from build123d import *

# Parameters (mm, degrees)
ESTRUSIONE_ESTRUSIONE1_DEPTH  = 10
TAGLIO_ESTRUSIONE1_DEPTH      = 3
SCHIZZO4_W                    = 80
SCHIZZO4_H                    = 5
ESTRUSIONE_ESTRUSIONE2_DEPTH  = 35
ESTRUSIONE_ESTRUSIONE4_DEPTH  = 80
SCHIZZO7_W                    = 80
SCHIZZO7_H                    = 5
ESTRUSIONE_ESTRUSIONE5_DEPTH  = 7
TAGLIO_ESTRUSIONE2_REACH      = 112.369
SCHIZZO8_R                    = 1.5
RACCORDO1_R                   = 5
RACCORDO2_R                   = 5
TAGLIO_ESTRUSIONE3_DEPTH      = 111.368700273
TAGLIO_ESTRUSIONE3_DEPTH_BACK = 10
SCHIZZO11_R                   = 4
TAGLIO_ESTRUSIONE4_DEPTH      = 3
SCHIZZO12_W                   = 12
SCHIZZO12_H                   = 12
ESTRUSIONE_ESTRUSIONE6_DEPTH  = 40
SCHIZZO13_R                   = 1.5
TAGLIO_ESTRUSIONE5_DEPTH      = 111.368700273
SCHIZZO14_R                   = 4
TAGLIO_ESTRUSIONE6_DEPTH      = 10


with BuildPart() as part:
    # Schizzo1 → Estrusione-Estrusione1 (new body)
    with BuildSketch(Plane.XY):
        with BuildLine():
            Line((-76.016095604, 20), (76.016095604, 20))
            ThreePointArc((76.016095604, 20), (92.5, 0), (76.016095604, -20))
            Line((76.016095604, -20), (-76.016095604, -20))
            ThreePointArc((-76.016095604, -20), (-92.5, 0), (-76.016095604, 20))
        make_face()
    extrude(amount=ESTRUSIONE_ESTRUSIONE1_DEPTH)

    # Schizzo3 → Taglio-Estrusione1 (cut)
    with BuildSketch(Plane.XY.offset(10)):
        with BuildLine():
            Line((-75.5, -15), (75.5, -15))
            ThreePointArc((75.5, -15), (87.5, 0), (75.5, 15))
            Line((75.5, 15), (-75.5, 15))
            ThreePointArc((-75.5, 15), (-87.5, 0), (-75.5, -15))
        make_face()
    extrude(amount=-TAGLIO_ESTRUSIONE1_DEPTH, mode=Mode.SUBTRACT)

    # Schizzo4 → Estrusione-Estrusione2 (add)
    with BuildSketch(Plane.XY.offset(10)):
        with Locations((0, -17.5)):
            Rectangle(SCHIZZO4_W, SCHIZZO4_H)
    estrusione_estrusione2 = extrude(amount=ESTRUSIONE_ESTRUSIONE2_DEPTH)

    # Schizzo6 → Estrusione-Estrusione4 (add)
    with BuildSketch(Plane(origin=(40, 0, 0), x_dir=(0, 0, -1), z_dir=(1, 0, 0))):
        Polygon((-40, -15), (-40, -12.81), (-7, -15), align=None)
    estrusione_estrusione4 = extrude(amount=-ESTRUSIONE_ESTRUSIONE4_DEPTH)

    # Schizzo7 → Estrusione-Estrusione5 (add)
    with BuildSketch(Plane(origin=(0, -15, 0), x_dir=(1, 0, 0), z_dir=(0, 1, 0))):
        with Locations((0, -42.5)):
            Rectangle(SCHIZZO7_W, SCHIZZO7_H)
    estrusione_estrusione5 = extrude(amount=ESTRUSIONE_ESTRUSIONE5_DEPTH)

    # Taglio-Estrusione2: up to this plane
    taglio_estrusione2_end = Plane(origin=(-40, -12.81, 40), z_dir=(1.4576135341627736e-15, 0.9978051809344605, -0.0662179801892863))
    # Schizzo8 → Taglio-Estrusione2 (cut, up to the surface)
    with BuildSketch(Plane.XZ.offset(20), mode=Mode.PRIVATE) as taglio_estrusione2_sk1:
        with Locations(Location((-30, 13, 0), (0, 0, 270))):
            Circle(SCHIZZO8_R)
    taglio_estrusione2_tool1 = split(extrude(taglio_estrusione2_sk1.sketch, amount=-TAGLIO_ESTRUSIONE2_REACH, mode=Mode.PRIVATE), bisect_by=taglio_estrusione2_end, keep=Keep.BOTH, mode=Mode.PRIVATE)
    add(taglio_estrusione2_tool1.solids().sort_by_distance((-30, -20, 13))[0], mode=Mode.SUBTRACT)
    # Schizzo8 → Taglio-Estrusione2 (cut, up to the surface)
    with BuildSketch(Plane.XZ.offset(20), mode=Mode.PRIVATE) as taglio_estrusione2_sk2:
        with Locations(Location((-30, 32, 0), (0, 0, 270))):
            Circle(SCHIZZO8_R)
    taglio_estrusione2_tool2 = split(extrude(taglio_estrusione2_sk2.sketch, amount=-TAGLIO_ESTRUSIONE2_REACH, mode=Mode.PRIVATE), bisect_by=taglio_estrusione2_end, keep=Keep.BOTH, mode=Mode.PRIVATE)
    add(taglio_estrusione2_tool2.solids().sort_by_distance((-30, -20, 32))[0], mode=Mode.SUBTRACT)
    # Schizzo8 → Taglio-Estrusione2 (cut, up to the surface)
    with BuildSketch(Plane.XZ.offset(20), mode=Mode.PRIVATE) as taglio_estrusione2_sk3:
        with Locations(Location((30, 13, 0), (0, 0, 270))):
            Circle(SCHIZZO8_R)
    taglio_estrusione2_tool3 = split(extrude(taglio_estrusione2_sk3.sketch, amount=-TAGLIO_ESTRUSIONE2_REACH, mode=Mode.PRIVATE), bisect_by=taglio_estrusione2_end, keep=Keep.BOTH, mode=Mode.PRIVATE)
    add(taglio_estrusione2_tool3.solids().sort_by_distance((30, -20, 13))[0], mode=Mode.SUBTRACT)
    # Schizzo8 → Taglio-Estrusione2 (cut, up to the surface)
    with BuildSketch(Plane.XZ.offset(20), mode=Mode.PRIVATE) as taglio_estrusione2_sk4:
        with Locations(Location((30, 32, 0), (0, 0, 270))):
            Circle(SCHIZZO8_R)
    taglio_estrusione2_tool4 = split(extrude(taglio_estrusione2_sk4.sketch, amount=-TAGLIO_ESTRUSIONE2_REACH, mode=Mode.PRIVATE), bisect_by=taglio_estrusione2_end, keep=Keep.BOTH, mode=Mode.PRIVATE)
    add(taglio_estrusione2_tool4.solids().sort_by_distance((30, -20, 32))[0], mode=Mode.SUBTRACT)

    # Specchia1: Estrusione-Estrusione2, Estrusione-Estrusione4, Estrusione-Estrusione5 across plane
    add(estrusione_estrusione2.mirror(Plane.ZX))
    add(estrusione_estrusione4.mirror(Plane.ZX))
    add(estrusione_estrusione5.mirror(Plane.ZX))

    # Raccordo1
    raccordo1_edges = [part.edges().sort_by_distance(p)[0] for p in [
        (0, -20, 45),
    ]]
    fillet(raccordo1_edges, radius=RACCORDO1_R)

    # Raccordo2
    raccordo2_edges = [part.edges().sort_by_distance(p)[0] for p in [
        (0, 20, 45),
    ]]
    fillet(raccordo2_edges, radius=RACCORDO2_R)

    # Schizzo9 → Taglio-Estrusione3 (cut, two sides)
    with BuildSketch(Plane.XZ.offset(20)) as taglio_estrusione3_sk:
        Polygon((-4, 11), (-4, 3), (4, 3), (4, 11), (10, 11), (10, 31), (-10, 31), (-10, 11), align=None)
    extrude(amount=TAGLIO_ESTRUSIONE3_DEPTH, mode=Mode.SUBTRACT)
    extrude(taglio_estrusione3_sk.sketch, amount=-TAGLIO_ESTRUSIONE3_DEPTH_BACK, mode=Mode.SUBTRACT)

    # Schizzo11 → Taglio-Estrusione4 (cut)
    with BuildSketch(Plane(origin=(0, -15.396736192, 1.021783402), x_dir=(1, 0, 0), z_dir=(1.4576135341627738e-15, 0.9978051809344605, -0.06621798018928632))):
        with Locations(Location((-30, -12.004564445, 0), (0, 0, 270))):
            Circle(SCHIZZO11_R)
        with Locations(Location((-30, -31.046357736, 0), (0, 0, 270))):
            Circle(SCHIZZO11_R)
        with Locations(Location((30, -31.046357736, 0), (0, 0, 270))):
            Circle(SCHIZZO11_R)
        with Locations(Location((30, -12.004564445, 0), (0, 0, 270))):
            Circle(SCHIZZO11_R)
    extrude(amount=-TAGLIO_ESTRUSIONE4_DEPTH, mode=Mode.SUBTRACT)

    # Schizzo12 → Estrusione-Estrusione6 (add)
    with BuildSketch(Plane.XZ.offset(20)):
        with Locations((70.016095604, -6)):
            Rectangle(SCHIZZO12_W, SCHIZZO12_H)
        with Locations((-70.016095604, -6)):
            Rectangle(SCHIZZO12_W, SCHIZZO12_H)
        with Locations((0, -6)):
            Rectangle(SCHIZZO12_W, SCHIZZO12_H)
    extrude(amount=-ESTRUSIONE_ESTRUSIONE6_DEPTH)

    # Schizzo13 → Taglio-Estrusione5 (cut, through all)
    with BuildSketch(Plane.XZ.offset(20)):
        with Locations(Location((-70.016095604, -6, 0), (0, 0, 270))):
            Circle(SCHIZZO13_R)
        with Locations(Location((0, -6, 0), (0, 0, 270))):
            Circle(SCHIZZO13_R)
        with Locations(Location((70.016095604, -6, 0), (0, 0, 270))):
            Circle(SCHIZZO13_R)
    extrude(amount=-TAGLIO_ESTRUSIONE5_DEPTH, mode=Mode.SUBTRACT)

    # Schizzo14 → Taglio-Estrusione6 (cut)
    with BuildSketch(Plane.XZ.offset(20)):
        with Locations(Location((-70.016095604, -6, 0), (0, 0, 270))):
            Circle(SCHIZZO14_R)
        with Locations(Location((0, -6, 0), (0, 0, 270))):
            Circle(SCHIZZO14_R)
        with Locations(Location((70.016095604, -6, 0), (0, 0, 270))):
            Circle(SCHIZZO14_R)
    taglio_estrusione6 = extrude(amount=-TAGLIO_ESTRUSIONE6_DEPTH, mode=Mode.SUBTRACT)

    # Specchia2: Taglio-Estrusione6 across plane
    add(taglio_estrusione6.mirror(Plane.ZX), mode=Mode.SUBTRACT)

    # TaglioSuperficie1
    split(bisect_by=Plane(origin=(0, 0, 0), x_dir=(1, 0, 0), z_dir=(0, 1, 0)), keep=Keep.BOTTOM)


solid = part.part
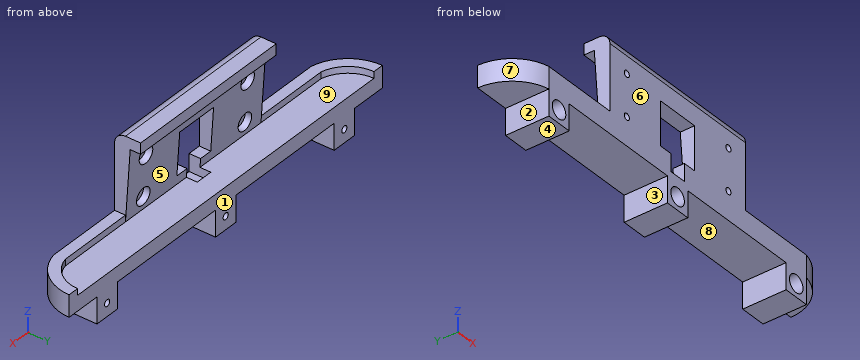
Work out the finished part from the listing and answer in its coordinate system (mm). Face numbers are marked on the shaded views. A direction names the side the tool comes from. Round coordinates to 2 decimals unless told otherwise and drop trailing zeros. Write each loop counter-clockwise with the first axis right and the second up, starting at its lowest first coordinate (ties: lowest second). Pieces come first, ordered by that corner, then holes.
1) A tool of negligible diameter and unlimited length cuts with its end or side. For the marked faces 1, 2, 3, 4 and 5, from which of +Z, -Z, +X, -X, +Y, -Y can it reach the whole face along a straight path? Write none if from no direction.
2) Straight lines are drawn through the part: line 1 (X direction, y = -13.75, z = -6); line 2 (X direction, y = -17.95, z = 32); line 3 (X direction, y = -19, z = 21.5). For each, find the intervals that lie inside material, in ascending order.
3) A cutting plane is placed at C-C (z = 38). Give the vertices of the cut face in (x, y), plus the area to 3 significant figures.
4) A cutting plane is placed at B-B (y = -5.25). Give the vertices of the cut face in (x, z), plus the area to 3 significant figures.
5) Given pin 1 Ø1.5 at (x, z) = (-49.5, 8) entering from +Y; pin 2 Ø10 at (x, y) = (-34.5, -7.5) entering from -Z; pin 3 Ø9 at (y, z) = (-16.5, 9) entering from -X; pin 4 Ø2.5 at (x, z) = (30, 32) entering from +Y, each flat-ended and moving along its own axis, determine where each tip first touches the part or whether it passes through.
6) A cutting plane is placed at A-A (x = 38). Give the vertices of the cut face in (y, z), plus the area to 3 significant figures.
7) The mould has two halves that part along X. Classify the marked faces 6, 7, 8 and 9: pulls with the +X half, pulls with the -X half, needs draft (parallel to the pull), parting line crosses it, or undercut.
Completed:
1. face 1: +Z, -Z, +X, -X, +Y
1. face 2: -Z, -X, +Y, -Y
1. face 3: -Z, +Y, -Y
1. face 4: -Z, +X, -X, +Y, -Y
1. face 5: +Y
2. line 1: x = -76.02 to -74.02, -66.02 to -64.02, -6 to -4, 4 to 6, 64.02 to 66.02, 74.02 to 76.02
2. line 2: x = -40 to -31.5, -28.5 to 28.5, 31.5 to 40
2. line 3: x = -40 to -10, 10 to 40
3. outline: (-40, -20) - (40, -20) - (40, -12.94) - (-40, -12.94) - close
3. area: 565 mm2
4. outline: (-91.81, 0) - (-76.02, 0) - (-76.02, -12) - (-64.02, -12) - (-64.02, 0) - (-6, 0) - (-6, -12) - (6, -12) - (6, 0) - (64.02, 0) - (64.02, -12) - (76.02, -12) - (76.02, 0) - (91.81, 0) - (91.81, 10) - (86.58, 10) - (86.58, 7) - (-86.58, 7) - (-86.58, 10) - (-91.81, 10) - close; hole circle Ø3 at (-70.02, -6); hole circle Ø3 at (0, -6); hole circle Ø3 at (70.02, -6)
4. area: 1,730 mm2
5. pin 1: stops at y = -15
5. pin 2: stops at z = 0
5. pin 3: stops at x = -88.59
5. pin 4: passes through
6. outline: (-20, 0) - (0, 0) - (0, 7) - (-15, 7) - (-12.81, 40) - (-8, 40) - (-8, 45) - (-15, 45) arc R5 ccw to (-20, 40) - close
6. area: 396 mm2
7. face 6: needs draft
7. face 7: pulls with the -X half
7. face 8: undercut
7. face 9: undercut
